Here's how the part is built. I have some questions about the finished solid (model axes, mm). Give positions to 0.01 mm unless a question says otherwise; leave off trailing zeros. Order: outer loops, then holes, each group sorted by start corner. A loop starts at its lowest first (then second) coordinate and runs counter-clockwise, first axis right, second up. Notation, with made-up numbers: (21, 5) -> (61, 5) arc R24 ccw to (61, 22) -> close; hole circle Ø8 at (14.5, 1). An arc over 180 degrees is marked (long way). Write each question's results on one line, items separated by ' | '. Start each with the question number.
Q1. I need wall thicknesses on line 1 along Y through (x, z) = (0, -14); line 2 along Z through (x, y) = (74, -17); line 3 along X through (y, z) = (2.5, 2.5). Which ranges of each line are inside material? Lowest first, please. Write a range as [from, to].
Q2. Imagine slicing it at A-A, the plane y = 0. Please give me the cut outline in (x, z).
Q3. Imagine slicing it at D-D, the plane y = 90. Please give me the cut outline in (x, z).
Q4. I'm going to push flat-ended pins straight in: pin 1 (10 mm diameter, centred on x = 25.5, y = -43.5, fed in from +Z); pin 2 (5.5 mm diameter, centred on x = 0, y = 0, fed in from -Z); pin 3 (6 mm diameter, centred on x = 2, y = 2, fed in from +Z). Where does each tip first touch, or does it pass through?
Q5. Imagine slicing it at C-C, the plane x = 23. Please give me the cut outline in (y, z).
Q6. Imagine slicing it at B-B, the plane z = -4. Please give me the cut outline in (x, y), then the cut area to 3 significant figures.
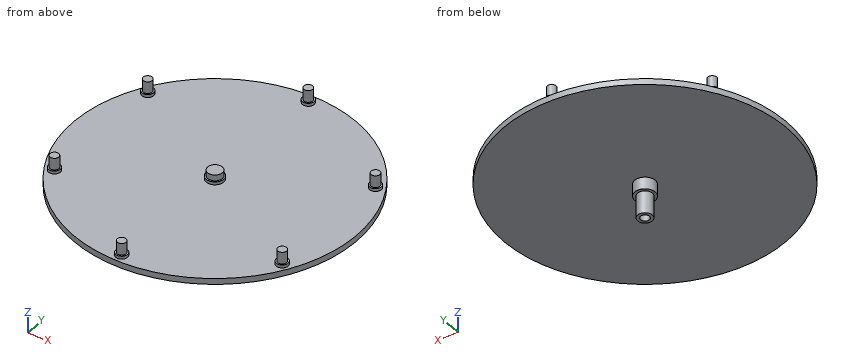
```python
from build123d import *

# Parameters (mm, degrees)
SKETCH_1_R               = 96
EXTRUDE_1_DEPTH          = 4
SKETCH_2_R               = 5
EXTRUDE_2_DEPTH          = 6
SKETCH_3_R               = 3
EXTRUDE_3_DEPTH          = 10
PATTERN_CIRCULAR_1_COUNT = 6
SKETCH_4_R               = 6
EXTRUDE_4_DEPTH          = 2
SKETCH_5_R               = 4
EXTRUDE_5_DEPTH          = 2
PATTERN_CIRCULAR_2_COUNT = 6
SKETCH_6_R               = 7
EXTRUDE_6_DEPTH          = 8
EXTRUDE_START            = 15
SKETCH_7_R               = 5
SKETCH_7_R_2             = 3
EXTRUDE_1_2_DEPTH        = 15


with BuildPart() as part:
    # 草图1 → Extrude 1 (new body)
    with BuildSketch(Plane.XY):
        Circle(SKETCH_1_R)
    extrude(amount=EXTRUDE_1_DEPTH)

    # 草图2 → 凸台-拉伸2 (add)
    with BuildSketch(Plane.XY.offset(4)):
        Circle(SKETCH_2_R)
    extrude(amount=EXTRUDE_2_DEPTH)

    # 草图3 → 凸台-拉伸3 (add)
    with BuildSketch(Plane.XY.offset(4)):
        with Locations((0, 90)):
            Circle(SKETCH_3_R)
    extrude_3 = extrude(amount=EXTRUDE_3_DEPTH)

    # 阵列(圆周)1: 凸台-拉伸3 ×6 about axis
    pattern_circular_1_axis = Axis((0, 0, 0), (0, 0, 1))
    for i in range(1, PATTERN_CIRCULAR_1_COUNT):
        add(extrude_3.rotate(pattern_circular_1_axis, i * 360 / PATTERN_CIRCULAR_1_COUNT))

    # 草图4 → 凸台-拉伸4 (add)
    with BuildSketch(Plane.XY.offset(4)):
        Circle(SKETCH_4_R)
    extrude(amount=EXTRUDE_4_DEPTH)

    # 草图5 → 凸台-拉伸5 (add)
    with BuildSketch(Plane.XY.offset(4)):
        with Locations((0, 90)):
            Circle(SKETCH_5_R)
    extrude_5 = extrude(amount=EXTRUDE_5_DEPTH)

    # 阵列(圆周)2: 凸台-拉伸5 ×6 about axis
    pattern_circular_2_axis = Axis((0, 0, 0), (0, 0, 1))
    for i in range(1, PATTERN_CIRCULAR_2_COUNT):
        add(extrude_5.rotate(pattern_circular_2_axis, i * 360 / PATTERN_CIRCULAR_2_COUNT))

    # 草图6 → 凸台-拉伸6 (add)
    with BuildSketch(Plane(origin=(0, 0, 0), x_dir=(-1, 0, 0), z_dir=(0, 0, -1))):
        with Locations(Location((0, 0, 0), (0, 0, 180))):
            Circle(SKETCH_6_R)
    extrude(amount=EXTRUDE_6_DEPTH)

    # 草图7 → Extrude 1 2 (add)
    with BuildSketch(Plane(origin=(0, 0, -8), x_dir=(-1, 0, 0), z_dir=(0, 0, -1)).offset(EXTRUDE_START)):
        Circle(SKETCH_7_R)
        Circle(SKETCH_7_R_2, mode=Mode.SUBTRACT)
    extrude(amount=-EXTRUDE_1_2_DEPTH)


solid = part.part
```
Geometry check:
1) line 1: [-5, -3], [3, 5] | line 2: [0, 4] | line 3: [-95.97, 95.97]
2) outline: (-96, 0) -> (-7, 0) -> (-7, -8) -> (-5, -8) -> (-5, -23) -> (-3, -23) -> (-3, -8) -> (3, -8) -> (3, -23) -> (5, -23) -> (5, -8) -> (7, -8) -> (7, 0) -> (96, 0) -> (96, 4) -> (6, 4) -> (6, 6) -> (5, 6) -> (5, 10) -> (-5, 10) -> (-5, 6) -> (-6, 6) -> (-6, 4) -> (-96, 4) -> close
3) outline: (-33.41, 0) -> (33.41, 0) -> (33.41, 4) -> (4, 4) -> (4, 6) -> (3, 6) -> (3, 14) -> (-3, 14) -> (-3, 6) -> (-4, 6) -> (-4, 4) -> (-33.41, 4) -> close
4) pin 1: z = 4 | pin 2: z = -8 | pin 3: z = 10
5) outline: (-93.2, 0) -> (93.2, 0) -> (93.2, 4) -> (-93.2, 4) -> close
6) outline: circle Ø14 at (0, 0) | area: 154 mm²
